```python
from build123d import *

# Parameters (mm, degrees)
F0_R     = 35.5
F0_R_2   = 33.5
F1_DEPTH = 50.8
F3_DEPTH = 50.8
F4_R     = 10
F5_DEPTH = 50.8
F7_DEPTH = 38.1


with BuildPart() as f1:
    # F0 (on Front) → F1 (new body)
    with BuildSketch(Plane.XZ):
        Circle(F0_R)
        Circle(F0_R_2, mode=Mode.SUBTRACT)
    extrude(amount=F1_DEPTH)

    # F2 (on Top) → F3 (cut)
    with BuildSketch(Plane.XY):
        with BuildLine():
            ThreePointArc((-6.457068, -22.28746), (23.128884, -25.78746), (-6.457068, -29.28746))
            Line((-6.457068, -29.28746), (-13.500003, -29.28746))
            Line((-13.500003, -29.28746), (-17.234227, -29.28746))
            Line((-17.234227, -29.28746), (-17.234227, -36.550397))
            Line((-17.234227, -36.550397), (-23.171365, -36.550397))
            Line((-23.171365, -36.550397), (-23.171365, -29.28746))
            Line((-23.171365, -29.28746), (-37.299089, -29.28746))
            Line((-37.299089, -29.28746), (-37.299089, -59.553057))
            Line((-37.299089, -59.553057), (42.624012, -59.553057))
            Line((42.624012, -59.553057), (42.624012, 5.546404))
            Line((42.624012, 5.546404), (-37.299089, 5.546404))
            Line((-37.299089, 5.546404), (-37.099175, -22.28746))
            Line((-37.099175, -22.28746), (-23.171365, -22.28746))
            Line((-23.171365, -22.28746), (-23.171365, -15.024522))
            Line((-23.171365, -15.024522), (-17.234227, -15.024522))
            Line((-17.234227, -15.024522), (-17.234227, -22.28746))
            Line((-17.234227, -22.28746), (-13.500003, -22.28746))
            Line((-13.500003, -22.28746), (-10.810506, -22.28746))
            Line((-10.810506, -22.28746), (-6.457068, -22.28746))
        make_face()
    extrude(amount=-F3_DEPTH, mode=Mode.SUBTRACT)

    # F4 (on Top) → F5 (cut)
    with BuildSketch(Plane.XY):
        with Locations((8.270558, -25.735088)):
            Circle(F4_R)
    extrude(amount=-F5_DEPTH, mode=Mode.SUBTRACT)

    # F6 (on Right) → F7 (cut, symmetric)
    with BuildSketch(Plane.YZ):
        Polygon((-21.942101, 38.113631), (-21.942101, 0), (-21.942101, -4.419958), (6.513468, -3.371595), (6.513468, 37.065268), align=None)
        Polygon((-29.430408, 0), (-29.430408, 39.161991), (-57.436682, 38.113631), (-57.436682, 0), align=None)
    extrude(amount=F7_DEPTH, both=True, mode=Mode.SUBTRACT)


solid = f1.part
```
Work out the finished part from the listing and answer in its coordinate system (mm). A direction names the side the tool comes from. Coordinates: 2 decimals unless noted, no trailing zeros. Order: outer loops, then holes, each group sorted by start corner. A loop starts at its lowest first (then second) coordinate and runs counter-clockwise, first axis right, second up. Notation, with made-up numbers: M -2.75,13.5 L 26.25,13.5 A12 cw 26.25,31.5 Z; hole C -7,-24 d7. An arc over 180 degrees is marked long. Use CSV: the item, a comma, the result in double quotes.
1) For faces 4 (the face through (-12, -29.287, -32)), 5 (the face through (19.985, -16.598, -29.008)), 6 (the face through (-12, -22.287, -32)), determine the directions among +Z, -Z, +X, -X, +Y, -Y from which every point of the face is accessible in a straight line to the end or side of a thin tool.
Worked out:
face 4,"-Z, -Y"
face 5,"-Z"
face 6,"-Z, +Y"
2) Consider line 1 (X direction, y = -33, z = -25); line 2 (Y direction, x = -17, z = -31); line 3 (X direction, y = -26, z = -1). Determine where each line is inside the solid, lowest interval first. Write a range as [from, to].
Worked out:
line 1,"x = [-23.17, -22.3]"
line 2,"y = [-29.29, -22.29]"
line 3,"x = [-35.49, -33.49]"
3) Section A-A on x = 4.5 is taken. Write down the section's boundary in (y, z).
Worked out:
outline,"M -40.34,-35.21 L -35,-35.21 L -35,-33.2 L -40.34,-33.2 Z; M -29.43,33.2 L -21.94,33.2 L -21.94,35.21 L -29.43,35.21 Z; M -16.47,-35.21 L -11.23,-35.21 L -11.23,-33.2 L -16.47,-33.2 Z"
4) Flat-ended cylindrical pins translate along their axes: pin 1 Ø6 at (x, z) = (-28.5, -11) entering from -Y; pin 2 Ø2 at (x, y) = (-5.5, -31) entering from -Z; pin 3 Ø1 at (x, y) = (-12, -22.5) entering from +Z. Find the tip coordinate at first contact, or state that the pin passes through.
Worked out:
pin 1,"stops at y = -29.29"
pin 2,"stops at z = -35.21"
pin 3,"stops at z = 33.59"
5) Section C-C on z = 15.5 is taken. Write down the section's boundary in (x, y).
Worked out:
outline,"M -31.94,-29.43 L -29.7,-29.43 L -29.7,-21.94 L -31.94,-21.94 Z; M 29.7,-29.43 L 31.94,-29.43 L 31.94,-21.94 L 29.7,-21.94 Z"
6) Section D-D on y = -24 is taken. Write down the section's boundary in (x, z).
Worked out:
outline,"M -1.58,-35.46 L -1.58,-33.46 A33.5 cw long 33.5,0 L 35.5,0 A35.5 ccw long Z; M 18.12,-30.53 A35.5 ccw 23.02,-27.02 L 23.02,-24.34 A33.5 cw 18.12,-28.18 Z"
7) Section B-B on y = -30.5 is taken. Write down the section's boundary in (x, z), plus the area to 3 significant figures.
Worked out:
outline,"M -23.17,-26.89 A35.5 ccw -17.23,-31.04 L -17.23,-28.73 A33.5 cw -23.17,-24.19 Z; M -6.11,-34.97 A35.5 ccw -0.52,-35.5 L -0.52,-33.5 A33.5 cw -6.11,-32.94 Z; M 17.06,-31.13 A35.5 ccw 22.37,-27.57 L 22.37,-24.94 A33.5 cw 17.06,-28.83 Z"
area,"39.0 mm^2"
8) Determine the mould class of faces 1 (the face through (-23.171, -33, -26)), 2 (the face through (15.239, -18.563, -31.774)), 3 (the face through (-5.1, -29.43, 33.4)) for opening direction X: released by +X, released by -X, zero draft, split by the parting line, or undercut.
Worked out:
face 1,"released by -X"
face 2,"undercut"
face 3,"zero draft"
